```python
from build123d import *

# Parameters (mm, degrees)
F0_W      = 30
F0_H      = 12
F1_DEPTH  = 15
F2_W      = 30
F2_H      = 1
F3_DEPTH  = 2.5
F4_W      = 30
F4_H      = 1
F5_DEPTH  = 2.5
F6_R      = 2.5
F7_DEPTH  = 15.001
F9_DEPTH  = 6
F10_R     = 6.5
F11_DEPTH = 2


# Not quite as in the source:
# - a feature names something its author has since deleted; it is built from what else it names


with BuildPart() as f1:
    # F0 (on Front) → F1 (new body)
    with BuildSketch(Plane.XZ):
        Rectangle(F0_W, F0_H)
    extrude(amount=F1_DEPTH)

    # F2 (on face) → F3 (join)
    with BuildSketch(Plane(origin=(0, 0, 0), x_dir=(-1, 0, 0), z_dir=(0, 1, 0))):
        with Locations((0, 6.5)):
            Rectangle(F2_W, F2_H)
        with BuildLine():
            ThreePointArc((15, 7), (0, 22), (-15, 7))
            Line((-15, 7), (15, 7))
        make_face()
    extrude(amount=-F3_DEPTH)

    # F4 (on face) → F5 (join)
    with BuildSketch(Plane.XZ.offset(15)):
        with Locations((0, 6.5)):
            Rectangle(F4_W, F4_H)
        with BuildLine():
            ThreePointArc((15, 7), (0, 22), (-15, 7))
            Line((-15, 7), (15, 7))
        make_face()
    extrude(amount=-F5_DEPTH)

    # F6 (on face) → F7 (cut, through all)
    with BuildSketch(Plane.XZ.offset(15)):
        with Locations((-1.01e-08, 17)):
            Circle(F6_R)
    extrude(amount=-F7_DEPTH, mode=Mode.SUBTRACT)

    # F8 (on face) → F9 (join)
    with BuildSketch(Plane(origin=(0, 0, -6), x_dir=(1, 0, 0), z_dir=(0, 0, -1))):
        with BuildLine():
            ThreePointArc((0, 0), (5.3033008589, 2.1966991411), (7.5, 7.5))
            ThreePointArc((7.5, 7.5), (5.3033008589, 12.8033008589), (0, 15))
            ThreePointArc((0, 15), (-7.5, 7.5), (0, 0))
        make_face()
    extrude(amount=F9_DEPTH)

    # F10 (on face) → F11 (cut)
    with BuildSketch(Plane(origin=(0, 0, -12), x_dir=(1, 0, 0), z_dir=(0, 0, -1))):
        with Locations((0, 7.5)):
            Circle(F10_R)
    extrude(amount=-F11_DEPTH, mode=Mode.SUBTRACT)


solid = f1.part
```
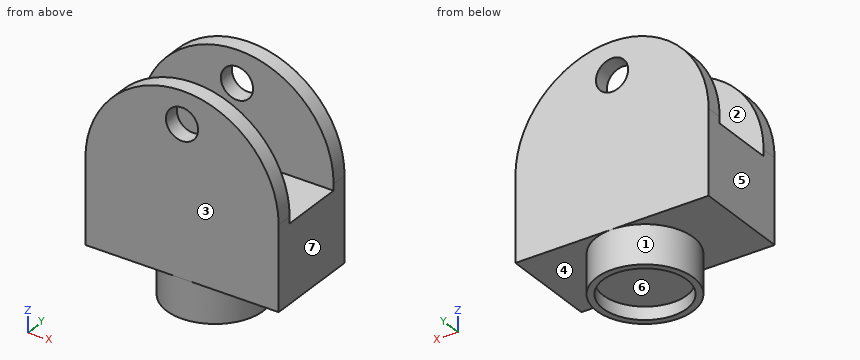
CAD build for the part. Positions are in the model's coordinates, mm. Face numbers are marked on the shaded views. A direction names the side the tool comes from. Round coordinates to 2 decimals unless told otherwise and drop trailing zeros. Loops run counter-clockwise (first coordinate to the right, second up) from the corner with the lowest first, then second, coordinate; pieces in that order, holes last. Notation, with made-up numbers: M 27,12.25 L 85,12.25 A19 ccw 85,26.25 Z; hole C 29.25,-14.75 d6. An arc over 180 degrees is marked long. Use a Markdown table: item, result. Add a question column.
(1) Flat gauge pins, fed straight in: pin 1 (2 mm diameter, centred on x = 11, y = -3, fed in from +Z); pin 2 (3 mm diameter, centred on x = 6.5, y = -5.5, fed in from +Z); pin 3 (8 mm diameter, centred on x = 0, z = 17, fed in from +Y); pin 4 (1.5 mm diameter, centred on y = -2.5, z = 10, fed in from +X). Where does each tip first touch, or does it go through?
(2) Cut at D-D (x = -9). Give the cut face in (y, z).
(3) Cut at A-A (y = -1.5). Give the cut face in (x, z), and give its area (3 significant figures).
(4) Which spindle directions (+Z, -Z, +X, -X, +Y, -Y) get a long thin tool onto all of the face, cutting with end or side? Do the marked faces 1, 2 and 3. Say none if no direction does.
(5) Drill centre lines: line 1 (Y direction, x = -10.5, z = 10); line 2 (X direction, y = -7.5, z = -11.5); line 3 (Z direction, x = -1, y = -11.75). Where is each one in solid material? Low to high.
(6) Cut at B-B (z = 18). Give the cut face in (x, y), and give its area (3 significant figures).
(7) Cut at C-C (z = 12.5). Give the cut face in (x, y).
(8) Pull direction X, two halves, no side cores. Call the marked faces 4, 5, 6 and 7: +X half, -X half, draft (parallel to the pull), parting line (faces both ways), or undercut.
Geometry says:
| question | item | result |
|---|---|---|
| 1 | pin 1 | stops at z = 18.06 |
| 1 | pin 2 | stops at z = 6 |
| 1 | pin 3 | stops at y = 0 |
| 1 | pin 4 | stops at x = 14.83 |
| 2 | outline | M -15,-6 L 0,-6 L 0,19 L -2.5,19 L -2.5,6 L -12.5,6 L -12.5,19 L -15,19 Z |
| 3 | outline | M -15,-6 L -4.5,-6 L -4.5,-12 L -2.5,-12 L -2.5,-10 L 2.5,-10 L 2.5,-12 L 4.5,-12 L 4.5,-6 L 15,-6 L 15,7 A15 ccw -15,7 Z; hole C 0,17 d5 |
| 3 | area | 768 mm² |
| 4 | face 1 | -Z |
| 4 | face 2 | +Z, +X, -X |
| 4 | face 3 | +Z, -Z, +X, -X, -Y |
| 5 | line 1 | y = -15 to -12.5, -2.5 to 0 |
| 5 | line 2 | x = -7.5 to -6.5, 6.5 to 7.5 |
| 5 | line 3 | z = -10 to 6 |
| 6 | outline | M -10.2,-15 L -2.29,-15 L -2.29,-12.5 L -10.2,-12.5 Z; M -10.2,-2.5 L -2.29,-2.5 L -2.29,0 L -10.2,0 Z; M 2.29,-15 L 10.2,-15 L 10.2,-12.5 L 2.29,-12.5 Z; M 2.29,-2.5 L 10.2,-2.5 L 10.2,0 L 2.29,0 Z |
| 6 | area | 79.1 mm² |
| 7 | outline | M -13.96,-15 L 13.96,-15 L 13.96,-12.5 L -13.96,-12.5 Z; M -13.96,-2.5 L 13.96,-2.5 L 13.96,0 L -13.96,0 Z |
| 8 | face 4 | draft |
| 8 | face 5 | -X half |
| 8 | face 6 | undercut |
| 8 | face 7 | +X half |
